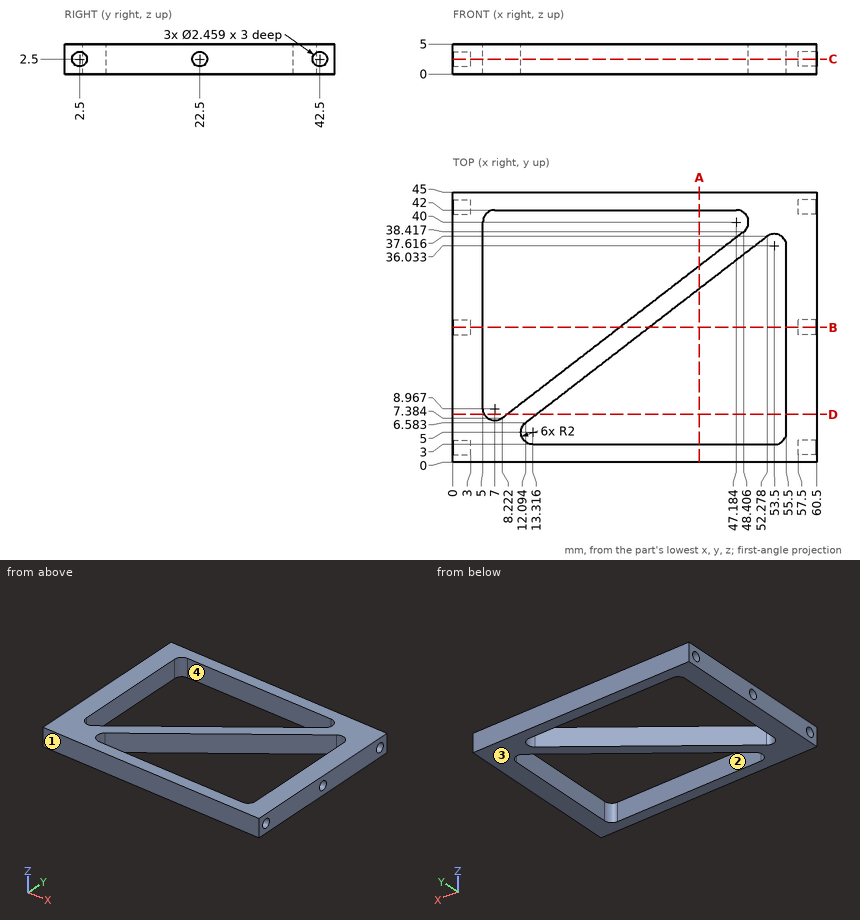
Design review of the part shown in the three views and the two pictorial views. Dimensions are in mm from the part's minimum x, y and z. A direction names the side the tool comes from. Coordinates: 2 decimals unless noted, no trailing zeros. Loops run counter-clockwise (first coordinate to the right, second up) from the corner with the lowest first, then second, coordinate; pieces in that order, holes last. Notation, with made-up numbers: M -35,88.5 L -1,88.5 A32 cw -1,122.5 Z; hole C 76,43.25 d5. An arc over 180 degrees is marked long. Put each result on its own line as item: value. Start each with the question number.
Q1. The part is to be moulded in two halves that separate along X. For the marked faces 3 and 4, say which applies: +X half, -X half, draft (parallel to the pull), parting line (faces both ways), or undercut.
Q2. Clearance check with flat-ended pins moving along their axes: pin 1 (3 mm diameter, centred on y = 42.5, z = 2.5, fed in from -X); pin 2 (0.7 mm diameter, centred on y = 23, z = 2.5, fed in from -X); pin 3 (1.2 mm diameter, centred on y = 3, z = 2.5, fed in from +X). State where each tip first meets the part, or that it passes through.
Q3. Add section D-D (y = 8). Write out the cut boundary in (x, z).
Q4. For the marked faces 1 and 2, list the 3-axis set-ups (+Z, -Z, +X, -X, +Y, -Y) from which the entire face can be reached by the end or side of a thin tool; tool diameter is ignored.
Q5. Add section A-A (x = 41). Write out the cut boundary in (y, z).
Q6. Wall thickness on line 1 (Y direction, x = 59.65, z = 2.5); line 2 (Z direction, x = 2.1, y = 2.5); line 3 (X direction, y = 30.5, z = 4.5) (1 decimal): over which ranges is each line inside the solid? List them lowest first.
Q7. Add section B-B (y = 22.5). Write out the cut boundary in (x, z) (1 decimal).
Q8. Add section C-C (z = 2.5). Count the separate pieces of the cut face and the enclosed holes in it.
Answers:
1. face 3: draft
1. face 4: undercut
2. pin 1: stops at x = 0
2. pin 2: stops at x = 3
2. pin 3: stops at x = 57.5
3. outline: M 0,0 L 5.25,0 L 5.25,5 L 0,5 Z; M 9.02,0 L 13.93,0 L 13.93,5 L 9.02,5 Z; M 55.5,0 L 60.5,0 L 60.5,5 L 55.5,5 Z
4. face 1: +Z, -Z, +X, -X, -Y
4. face 2: +Z, -Z
5. outline: M 0,0 L 3,0 L 3,5 L 0,5 Z; M 28.91,0 L 32.7,0 L 32.7,5 L 28.91,5 Z; M 42,0 L 45,0 L 45,5 L 42,5 Z
6. line 1: y = 0 to 1.27, 3.73 to 21.27, 23.73 to 41.27, 43.73 to 45
6. line 2: z = 0 to 1.27, 3.73 to 5
6. line 3: x = 0 to 5, 38.2 to 43.1, 55.5 to 60.5
7. outline: M 0,0 L 5,0 L 5,5 L 0,5 L 0,3.7 L 3,3.7 L 3,1.3 L 0,1.3 Z; M 27.8,0 L 32.7,0 L 32.7,5 L 27.8,5 Z; M 55.5,0 L 60.5,0 L 60.5,1.3 L 57.5,1.3 L 57.5,3.7 L 60.5,3.7 L 60.5,5 L 55.5,5 Z
8. separate pieces: 1
8. enclosed holes: 2
